from build123d import *

# Parameters (mm, degrees)
BOSS_EXTRUDE1_DEPTH = 38.1
SKETCH2_W           = 31.75
SKETCH2_H           = 31.75
CUT_EXTRUDE1_DEPTH  = 504.835943665


with BuildPart() as part:
    # Sketch1 → Boss-Extrude1 (new body)
    with BuildSketch(Plane(origin=(0, 0, 0), x_dir=(0, 0, -1), z_dir=(1, 0, 0))):
        with BuildLine():
            ThreePointArc((24.13, 19.05), (21.675298243, 8.446305074), (14.810617813, 0))
            Line((14.810617813, 0), (500.946542187, 0))
            ThreePointArc((500.946542187, 0), (491.62716, 19.05), (500.946542187, 38.1))
            Line((500.946542187, 38.1), (14.810617813, 38.1))
            ThreePointArc((14.810617813, 38.1), (21.675298243, 29.653694926), (24.13, 19.05))
        make_face()
    extrude(amount=BOSS_EXTRUDE1_DEPTH)

    # Sketch2 → Cut-Extrude1 (cut, through all)
    with BuildSketch(Plane.XY):
        with Locations((19.05, 19.05)):
            Rectangle(SKETCH2_W, SKETCH2_H)
    extrude(amount=-CUT_EXTRUDE1_DEPTH, mode=Mode.SUBTRACT)


solid = part.part
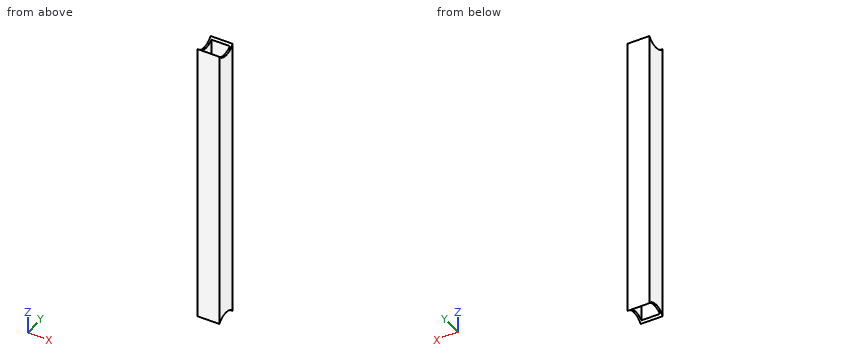
Input: part model. Units: mm. Frame: model coordinates. Coordinates: 2 decimals unless noted, no trailing zeros. Write each loop counter-clockwise with the first axis right and the second up, starting at its lowest first coordinate (ties: lowest second). Pieces come first, ordered by that corner, then holes. Notation, with made-up numbers: M 46,33 L 90,33 A21 cw 90,69 Z; hole C 56.25,-30.5 d9. An arc over 180 degrees is marked long. Answer as a JSON object with one key per item and string values. Group by question number.
(1) Section C-C on y = 11.5. Output: boundary loops of the cut face in (x, z) (3 decimals).
(2) Section A-A on z = -281.5. Output: boundary loops of the cut face in (x, y) (3 decimals), plus the area to 3 significant figures.
(3) Contact query for flat-ended pins moving along their axis: P1, Ø8, axis at x = 5.5, y = 16, coming from the +Z side; P2, Ø12, axis at x = 7, y = 24.5, coming from the -Z side; P3, Ø3, axis at x = 16, y = 6.5, coming from the +Z side; P4, Ø8, axis at x = 5.5, y = 10, coming from the -Z side. Output: stop coordinate, or through.
(4) Ray query, line 1 along X through (y, z) = (3.5, -133.5) (3 decimals); line 2 along Z through (x, y) = (2.5, 33). Return the intervals inside material, ascending. Write a range as [from, to].
(5) Section B-B on x = 15. Output: boundary loops of the cut face in (y, z) (3 decimals), plus the area to 3 significant figures.
Result set:
{
 "1": {"outline": "M 0,-492.839 L 3.175,-492.839 L 3.175,-22.918 L 0,-22.918 Z; M 34.925,-492.839 L 38.1,-492.839 L 38.1,-22.918 L 34.925,-22.918 Z"},
 "2": {"outline": "M 0,0 L 38.1,0 L 38.1,38.1 L 0,38.1 Z; hole M 3.175,3.175 L 34.925,3.175 L 34.925,34.925 L 3.175,34.925 Z", "area": "444 mm2"},
 "3": {"P1": "stops at z = -23.29", "P2": "stops at z = -493.83", "P3": "passes through", "P4": "stops at z = -495"},
 "4": {"line 1": "x = [0, 3.175], [34.925, 38.1]", "line 2": "z = [-496.07, -19.69]"},
 "5": {"outline": "M 0,-500.947 A24.13 cw 3.175,-497.585 L 3.175,-18.173 A24.13 cw 0,-14.811 Z; M 34.925,-497.585 A24.13 cw 38.1,-500.947 L 38.1,-14.811 A24.13 cw 34.925,-18.173 Z", "area": "3,060 mm2"}
}
